Here's how the part is built. I have some questions about the finished solid (model axes, mm). A direction names the side the tool comes from. Round coordinates to 2 decimals unless told otherwise and drop trailing zeros. Order: outer loops, then holes, each group sorted by start corner. A loop starts at its lowest first (then second) coordinate and runs counter-clockwise, first axis right, second up.
```python
from build123d import *

# Parameters (mm, degrees)
F1_R     = 22.70121
F2_DEPTH = 31.75
F0_W     = 57.163614
F0_H     = 30.503861
F3_DEPTH = 10.922
F4_R     = 16.805864
F5_DEPTH = 45.466
F6_W     = 22.098323
F6_H     = 9.037962
F7_DEPTH = 11.938
F9_DEPTH = 25.4


with BuildPart() as f2:
    # F1 (on face) → F2 (new body)
    with BuildSketch(Plane.XY):
        with Locations((-44.346001, -23.394492)):
            Circle(F1_R)
    extrude(amount=F2_DEPTH)

    # F0 (on Top) → F3 (join)
    with BuildSketch(Plane.XY):
        with Locations((-16.275043, -23.01623)):
            Rectangle(F0_W, F0_H)
    extrude(amount=F3_DEPTH)

    # F4 (on face) → F5 (cut)
    with BuildSketch(Plane.XY.offset(31.75)):
        with Locations((-44.346001, -23.394492)):
            Circle(F4_R)
    extrude(amount=-F5_DEPTH, mode=Mode.SUBTRACT)

    # F6 (on face) → F7 (join)
    with BuildSketch(Plane.XY.offset(10.922)):
        with Locations((-11.049162, -23.398413)):
            Rectangle(F6_W, F6_H)
    extrude(amount=F7_DEPTH)

    # F8 (on face) → F9 (cut)
    with BuildSketch(Plane(origin=(0, -18.879432, 0), x_dir=(-1, 0, 0), z_dir=(0, 1, 0))):
        Polygon((0, 10.922), (22.098323, 22.86), (0, 22.86), align=None)
    extrude(amount=-F9_DEPTH, mode=Mode.SUBTRACT)


solid = f2.part
```
1. I'm going to push flat-ended pins straight in: P1, Ø5.5, axis at x = -1, z = 3.5, coming from the -Y side; P2, Ø10, axis at y = -6.5, z = 16.5, coming from the -X side; P3, Ø13, axis at x = -8, z = 15, coming from the +Y side. Where does each tip first touch, or does it pass through?
Evaluation:
P1: stops at y = -38.27
P2: stops at x = -63.68
P3: stops at y = -7.76
2. If we section it at A-A, the plane y = -20: Write out the boundary of the cut face in (x, z).
Evaluation:
outline: (-66.79, 0) - (-60.81, 0) - (-60.81, 31.75) - (-66.79, 31.75) - close; (-27.89, 0) - (12.31, 0) - (12.31, 10.92) - (0, 10.92) - (-22.1, 22.86) - (-21.9, 22.86) - (-21.9, 31.75) - (-27.89, 31.75) - close
3. If we section it at D-D, the plane x = -4: Write out the boundary of the cut face in (y, z), and give its area (3 significant figures).
Evaluation:
outline: (-38.27, 0) - (-7.76, 0) - (-7.76, 10.92) - (-18.88, 10.92) - (-18.88, 13.08) - (-27.92, 13.08) - (-27.92, 10.92) - (-38.27, 10.92) - close
area: 353 mm2
4. If we mould it in two halves opening along Z, with no side actions, what happens to faces 1 (the flat face through (-19, -23, 0)), 2 (the cylindrical face through (-28.316, -18.346, 16.097)), 3 (the flat face through (1, -23, 10.922))? For each: released by +Z, released by -Z, zero draft, split by the parting line, or undercut.
Evaluation:
face 1: released by -Z
face 2: zero draft
face 3: released by +Z
5. I need wall thicknesses on probe 1 along Y at (x, z) = (-45, 7); probe 2 along Y at (x, z) = (-1.5, 6); probe 3 along X at (y, z) = (-36, 29). Which ranges of each line are inside material? Lowest first, please.
Evaluation:
probe 1: y = -46.09 to -40.19, -6.6 to -0.7
probe 2: y = -38.27 to -7.76
probe 3: x = -63.23 to -55.46, -33.23 to -25.47
6. On a 3-axis mill with a long thin cutter (end or side, diameter ignored), from which of +Z, -Z, +X, -X, +Y, -Y can I reach the whole of each face in a straight line? I mean faces 4 (the flat face through (-8, -38.268, 5)), 5 (the flat face through (-8, -7.764, 5)), 6 (the flat face through (-14, -18.879, 15)), 7 (the flat face through (-14, -27.917, 15)). Say none if no direction works.
Evaluation:
face 4: +Z, -Z, +X, -Y
face 5: +Z, -Z, +X, +Y
face 6: +Z, +X, +Y
face 7: +Z, +X, -Y
7. If we section it at B-B, the plane x = -44.5: Write out the boundary of the cut face in (y, z).
Evaluation:
outline: (-46.1, 0) - (-40.2, 0) - (-40.2, 31.75) - (-46.1, 31.75) - close; (-6.59, 0) - (-0.69, 0) - (-0.69, 31.75) - (-6.59, 31.75) - close
